```python
from build123d import *

# Parameters (mm, degrees)
F0_W      = 50
F0_H      = 50
F1_DEPTH  = 50
F2_R      = 5
F3_DEPTH  = 1
F4_R      = 5
F6_R      = 5
F7_DEPTH  = 1
F9_R      = 5
F10_DEPTH = 1
F12_R     = 5
F13_DEPTH = 1
F15_R     = 5
F16_DEPTH = 1
F18_R     = 5
F19_DEPTH = 1
F21_DEPTH = 0.5


# Not quite as in the source:
# - a fillet or chamfer that OpenCascade refuses, or shapes differently, is made with other operations: its cross-section is extruded or revolved along the edge and cut away or added
# - a feature names something its author has since deleted; it is built from what else it names


with BuildPart() as f1:
    # F0 (on Top) → F1 (new body)
    with BuildSketch(Plane.XY):
        with Locations((25, -25)):
            Rectangle(F0_W, F0_H)
    extrude(amount=F1_DEPTH)

    # F2 (on face) → F3 (cut)
    with BuildSketch(Plane.XY.offset(50)):
        with Locations((25, -25)):
            Circle(F2_R)
    extrude(amount=-F3_DEPTH, mode=Mode.SUBTRACT)

    # F4
    f4_edges = [f1.edges().sort_by_distance(p)[0] for p in [
        (0, -50, 25),
        (25, -50, 50),
        (25, 0, 50),
        (0, 0, 25),
        (0, -25, 0),
        (0, -25, 50),
        (25, -50, 0),
        (50, -50, 25),
        (25, 0, 0),
        (50, 0, 25),
        (50, -25, 0),
        (50, -25, 50),
    ]]
    fillet(f4_edges, radius=F4_R)

    # F5: fillet of radius 5 on 1 edges, made by hand

    # F5_s1 → F5_t2 (revolve)
    with BuildSketch(Plane.XZ.offset(25)):
        with BuildLine():
            ThreePointArc((30, 50), (28.5811388301, 49.2565835097), (27, 49))
            Line((27, 49), (30, 49))
            Line((30, 49), (30, 50))
        make_face()
    revolve(axis=Axis((25, -25, 49), (0, 0, 1)))

    # F6 (on face) → F7 (cut)
    with BuildSketch(Plane.XZ.offset(50)):
        with Locations((15, 35)):
            Circle(F6_R)
        with Locations((35, 35)):
            Circle(F6_R)
        with Locations((35, 15)):
            Circle(F6_R)
        with Locations((15, 15)):
            Circle(F6_R)
    extrude(amount=-F7_DEPTH, mode=Mode.SUBTRACT)

    # F8: fillet of radius 5 on 4 edges, made by hand

    # F8_s1 → F8_t2 (revolve)
    with BuildSketch(Plane.XY.offset(35)):
        with BuildLine():
            ThreePointArc((20, -50), (18.5811388301, -49.2565835097), (17, -49))
            Line((17, -49), (20, -49))
            Line((20, -49), (20, -50))
        make_face()
    revolve(axis=Axis((15, -49, 35), (0, -1, 0)))

    # F8_s3 → F8_t4 (revolve)
    with BuildSketch(Plane.XY.offset(35)):
        with BuildLine():
            ThreePointArc((40, -50), (38.5811388301, -49.2565835097), (37, -49))
            Line((37, -49), (40, -49))
            Line((40, -49), (40, -50))
        make_face()
    revolve(axis=Axis((35, -49, 35), (0, -1, 0)))

    # F8_s5 → F8_t6 (revolve)
    with BuildSketch(Plane.XY.offset(15)):
        with BuildLine():
            ThreePointArc((20, -50), (18.5811388301, -49.2565835097), (17, -49))
            Line((17, -49), (20, -49))
            Line((20, -49), (20, -50))
        make_face()
    revolve(axis=Axis((15, -49, 15), (0, -1, 0)))

    # F8_s7 → F8_t8 (revolve)
    with BuildSketch(Plane.XY.offset(15)):
        with BuildLine():
            ThreePointArc((40, -50), (38.5811388301, -49.2565835097), (37, -49))
            Line((37, -49), (40, -49))
            Line((40, -49), (40, -50))
        make_face()
    revolve(axis=Axis((35, -49, 15), (0, -1, 0)))

    # F9 (on face) → F10 (cut)
    with BuildSketch(Plane(origin=(0, 0, 0), x_dir=(-1, 0, 0), z_dir=(0, 1, 0))):
        with Locations((-35, 15)):
            Circle(F9_R)
        with Locations((-15, 35)):
            Circle(F9_R)
    extrude(amount=-F10_DEPTH, mode=Mode.SUBTRACT)

    # F11: fillet of radius 5 on 2 edges, made by hand

    # F11_s1 → F11_t2 (revolve)
    with BuildSketch(Plane.XY.offset(15)):
        with BuildLine():
            ThreePointArc((30, 0), (31.4188611699, -0.7434164903), (33, -1))
            Line((33, -1), (30, -1))
            Line((30, -1), (30, 0))
        make_face()
    revolve(axis=Axis((35, -1, 15), (0, 1, 0)))

    # F11_s3 → F11_t4 (revolve)
    with BuildSketch(Plane.XY.offset(35)):
        with BuildLine():
            ThreePointArc((10, 0), (11.4188611699, -0.7434164903), (13, -1))
            Line((13, -1), (10, -1))
            Line((10, -1), (10, 0))
        make_face()
    revolve(axis=Axis((15, -1, 35), (0, 1, 0)))

    # F12 (on face) → F13 (cut)
    with BuildSketch(Plane.YZ.offset(50)):
        with Locations((-15, 35)):
            Circle(F12_R)
        with Locations((-25, 25)):
            Circle(F12_R)
        with Locations((-35, 15)):
            Circle(F12_R)
    extrude(amount=-F13_DEPTH, mode=Mode.SUBTRACT)

    # F14: fillet of radius 5 on 3 edges, made by hand

    # F14_s1 → F14_t2 (revolve)
    with BuildSketch(Plane.XY.offset(15)):
        with BuildLine():
            ThreePointArc((50, -30), (49.2565835097, -31.4188611699), (49, -33))
            Line((49, -33), (49, -30))
            Line((49, -30), (50, -30))
        make_face()
    revolve(axis=Axis((49, -35, 15), (1, 0, 0)))

    # F14_s3 → F14_t4 (revolve)
    with BuildSketch(Plane.XY.offset(25)):
        with BuildLine():
            ThreePointArc((50, -20), (49.2565835097, -21.4188611699), (49, -23))
            Line((49, -23), (49, -20))
            Line((49, -20), (50, -20))
        make_face()
    revolve(axis=Axis((49, -25, 25), (1, 0, 0)))

    # F14_s5 → F14_t6 (revolve)
    with BuildSketch(Plane.XY.offset(35)):
        with BuildLine():
            ThreePointArc((50, -10), (49.2565835097, -11.4188611699), (49, -13))
            Line((49, -13), (49, -10))
            Line((49, -10), (50, -10))
        make_face()
    revolve(axis=Axis((49, -15, 35), (1, 0, 0)))

    # F15 (on face) → F16 (cut)
    with BuildSketch(Plane(origin=(0, 0, 0), x_dir=(0, -1, 0), z_dir=(-1, 0, 0))):
        with Locations((15, 35)):
            Circle(F15_R)
        with Locations((25, 25)):
            Circle(F15_R)
        with Locations((15, 15)):
            Circle(F15_R)
        with Locations((35, 15)):
            Circle(F15_R)
        with Locations((35, 35)):
            Circle(F15_R)
    extrude(amount=-F16_DEPTH, mode=Mode.SUBTRACT)

    # F17: fillet of radius 5 on 5 edges, made by hand

    # F17_s1 → F17_t2 (revolve)
    with BuildSketch(Plane.XY.offset(35)):
        with BuildLine():
            ThreePointArc((0, -20), (0.7434164903, -18.5811388301), (1, -17))
            Line((1, -17), (1, -20))
            Line((1, -20), (0, -20))
        make_face()
    revolve(axis=Axis((1, -15, 35), (-1, 0, 0)))

    # F17_s3 → F17_t4 (revolve)
    with BuildSketch(Plane.XY.offset(25)):
        with BuildLine():
            ThreePointArc((0, -30), (0.7434164903, -28.5811388301), (1, -27))
            Line((1, -27), (1, -30))
            Line((1, -30), (0, -30))
        make_face()
    revolve(axis=Axis((1, -25, 25), (-1, 0, 0)))

    # F17_s5 → F17_t6 (revolve)
    with BuildSketch(Plane.XY.offset(15)):
        with BuildLine():
            ThreePointArc((0, -40), (0.7434164903, -38.5811388301), (1, -37))
            Line((1, -37), (1, -40))
            Line((1, -40), (0, -40))
        make_face()
    revolve(axis=Axis((1, -35, 15), (-1, 0, 0)))

    # F17_s7 → F17_t8 (revolve)
    with BuildSketch(Plane.XY.offset(35)):
        with BuildLine():
            ThreePointArc((0, -40), (0.7434164903, -38.5811388301), (1, -37))
            Line((1, -37), (1, -40))
            Line((1, -40), (0, -40))
        make_face()
    revolve(axis=Axis((1, -35, 35), (-1, 0, 0)))

    # F17_s9 → F17_t10 (revolve)
    with BuildSketch(Plane.XY.offset(15)):
        with BuildLine():
            ThreePointArc((0, -20), (0.7434164903, -18.5811388301), (1, -17))
            Line((1, -17), (1, -20))
            Line((1, -20), (0, -20))
        make_face()
    revolve(axis=Axis((1, -15, 15), (-1, 0, 0)))

    # F18 (on face) → F19 (cut)
    with BuildSketch(Plane(origin=(0, 0, 0), x_dir=(1, 0, 0), z_dir=(0, 0, -1))):
        with Locations((15, 37)):
            Circle(F18_R)
        with Locations((15, 25)):
            Circle(F18_R)
        with Locations((15, 13)):
            Circle(F18_R)
        with Locations((35, 37)):
            Circle(F18_R)
        with Locations((35, 13)):
            Circle(F18_R)
        with Locations((35, 25)):
            Circle(F18_R)
    extrude(amount=-F19_DEPTH, mode=Mode.SUBTRACT)

    # F20: fillet of radius 5 on 6 edges, made by hand

    # F20_s1 → F20_t2 (revolve)
    with BuildSketch(Plane.XZ.offset(25)):
        with BuildLine():
            ThreePointArc((40, 0), (38.5811388301, 0.7434164903), (37, 1))
            Line((37, 1), (40, 1))
            Line((40, 1), (40, 0))
        make_face()
    revolve(axis=Axis((35, -25, 1), (0, 0, -1)))

    # F20_s3 → F20_t4 (revolve)
    with BuildSketch(Plane.XZ.offset(25)):
        with BuildLine():
            ThreePointArc((20, 0), (18.5811388301, 0.7434164903), (17, 1))
            Line((17, 1), (20, 1))
            Line((20, 1), (20, 0))
        make_face()
    revolve(axis=Axis((15, -25, 1), (0, 0, -1)))

    # F20_s5 → F20_t6 (revolve)
    with BuildSketch(Plane.XZ.offset(37)):
        with BuildLine():
            ThreePointArc((20, 0), (18.5811388301, 0.7434164903), (17, 1))
            Line((17, 1), (20, 1))
            Line((20, 1), (20, 0))
        make_face()
    revolve(axis=Axis((15, -37, 1), (0, 0, -1)))

    # F20_s7 → F20_t8 (revolve)
    with BuildSketch(Plane.XZ.offset(13)):
        with BuildLine():
            ThreePointArc((20, 0), (18.5811388301, 0.7434164903), (17, 1))
            Line((17, 1), (20, 1))
            Line((20, 1), (20, 0))
        make_face()
    revolve(axis=Axis((15, -13, 1), (0, 0, -1)))

    # F20_s9 → F20_t10 (revolve)
    with BuildSketch(Plane.XZ.offset(13)):
        with BuildLine():
            ThreePointArc((40, 0), (38.5811388301, 0.7434164903), (37, 1))
            Line((37, 1), (40, 1))
            Line((40, 1), (40, 0))
        make_face()
    revolve(axis=Axis((35, -13, 1), (0, 0, -1)))

    # F20_s11 → F20_t12 (revolve)
    with BuildSketch(Plane.XZ.offset(37)):
        with BuildLine():
            ThreePointArc((40, 0), (38.5811388301, 0.7434164903), (37, 1))
            Line((37, 1), (40, 1))
            Line((40, 1), (40, 0))
        make_face()
    revolve(axis=Axis((35, -37, 1), (0, 0, -1)))

    # F21 (add): a face of the model
    f21_faces = [f1.faces().sort_by_distance(p)[0] for p in [
        (25, -25, 0),
    ]]
    extrude(f21_faces, amount=-F21_DEPTH)


solid = f1.part
```
Check sheet for the modelled part. Datum: model origin and axes. Units: mm. A direction names the side the tool comes from. Round coordinates to 2 decimals unless told otherwise and drop trailing zeros. Order: outer loops, then holes, each group sorted by start corner. A loop starts at its lowest first (then second) coordinate and runs counter-clockwise, first axis right, second up. Notation, with made-up numbers: (-29.5, 4) -> (10.5, 4) arc R27 ccw to (10.5, 41) -> close; hole circle Ø10 at (-39, 57). An arc over 180 degrees is marked (long way). One line per item, written item: value. Start each with the question number.
Q1. Cross-section at B-B (y = -46). Record the boundary of the cut face in (x, z).
Q2. Cross-section at A-A (x = 3). Record the boundary of the cut face in (y, z).
Q3. Gauge pin test, flat ends, axial feed: pin 1 Ø4.5 at (x, z) = (35, 15.5) entering from +Y; pin 2 Ø1.2 at (x, y) = (25.5, -25.5) entering from +Z; pin 3 Ø2 at (x, z) = (16, 35) entering from +Y. Record the tip position at first contact, or that the pin passes through.
Q4. Set-up check for faces 4 (the face through (1, -35, 15)), 5 (the face through (49, -25, 25)), 6 (the face through (15, -49, 35)), 7 (the face through (35, -13, 1)): record each of +Z, -Z, +X, -X, +Y, -Y from which the full face is reachable in a straight line by a thin tool's end or side.
Q5. Thickness scan on line 1 (Z direction, x = 7, y = -48); line 2 (Z direction, x = 23, y = -24). Record the ranges inside material, lowest first.
Q6. Mould release check, pull along X, two halves, no side actions. Record for faces 1 (the face through (15, -1, 35)), 2 (the face through (25, -49, 48)), 3 (the face through (50, -30, 20)): pulls with the +X half, pulls with the -X half, needs draft (parallel to the pull), parting line crosses it, or undercut.
Completed:
1. outline: (0.1, 5) arc R4.9 ccw to (5, 0.1) -> (45, 0.1) arc R4.9 ccw to (49.9, 5) -> (49.9, 45) arc R4.9 ccw to (45, 49.9) -> (5, 49.9) arc R4.9 ccw to (0.1, 45) -> close
2. outline: (-49.58, 5) arc R4.58 ccw to (-45, 0.42) -> (-5, 0.42) arc R4.58 ccw to (-0.42, 5) -> (-0.42, 45) arc R4.58 ccw to (-5, 49.58) -> (-45, 49.58) arc R4.58 ccw to (-49.58, 45) -> close
3. pin 1: stops at y = -0.94
3. pin 2: stops at z = 49
3. pin 3: stops at y = -1
4. face 4: -X
4. face 5: +X
4. face 6: -Y
4. face 7: -Z
5. line 1: z = 1 to 49
5. line 2: z = 0 to 49.01
6. face 1: undercut
6. face 2: needs draft
6. face 3: pulls with the +X half
